```python
from build123d import *

# Parameters (mm, degrees)
F0_R     = 0.5
F1_DEPTH = 9
F2_W     = 3
F2_H     = 2
F3_DEPTH = 1.501


with BuildPart() as f1:
    # F0 (on Right) → F1 (new body)
    with BuildSketch(Plane.YZ):
        with BuildLine():
            ThreePointArc((0, 1.5), (-0.75, 0.75), (0, 0))
            Line((0, 0), (20, 0))
            ThreePointArc((20, 0), (20.75, 0.75), (20, 1.5))
            Line((20, 1.5), (0, 1.5))
        make_face()
        with Locations((0, 0.75)):
            Circle(F0_R, mode=Mode.SUBTRACT)
    extrude(amount=F1_DEPTH)

    # F2 (on Top) → F3 (cut, through all)
    with BuildSketch(Plane.XY):
        with Locations((1.5, 0.25)):
            Rectangle(F2_W, F2_H)
        with Locations((7.5, 0.25)):
            Rectangle(F2_W, F2_H)
    extrude(amount=F3_DEPTH, mode=Mode.SUBTRACT)


solid = f1.part
```
Work out the finished part from the listing and answer in its coordinate system (mm). A direction names the side the tool comes from. Give positions to 0.01 mm unless a question says otherwise; leave off trailing zeros. Loops run counter-clockwise (first coordinate to the right, second up) from the corner with the lowest first, then second, coordinate; pieces in that order, holes last. Notation, with made-up numbers: (-13.5, 83.5) -> (45.5, 83.5) arc R20 cw to (45.5, 100.5) -> close; hole circle Ø5 at (31.25, 11). An arc over 180 degrees is marked (long way). Write item = value, one per line. Start each with the question number.
(1) Find the intervals of material crossed by probe 1 along Y at (x, z) = (4.85, 0.75); probe 2 along Y at (x, z) = (6.25, 0.7); probe 3 along Y at (x, z) = (2.25, 0.35), in increasing order. Write a range as from..to.
(2) Which of the six approach directions +Z, -Z, +X, -X, +Y, -Y give full straight-line access (tool end or side, diameter ignored) to faces 1 (the flat face through (7, 1.25, 1)), 2 (the cylindrical face through (4.44, 20.75, 0.73)), 3 (the flat face through (3, 1, 1))?
(3) Find section A-A on z = 0.75. Give the vertices of the cut face in (x, y).
(4) The mould has two halves that part along Z. Classify faces 4 (the flat face through (6, 1, 1)), 5 (the cylindrical face through (4.479, -0.108, 0.262)), 6 (the flat face through (4, 10, 1.5)): +Z half, -Z half, draft (parallel to the pull), parting line (faces both ways), or undercut.
(5) Find section B-B on x = 2.25. Give the vertices of the cut face in (y, z), and give its area (3 significant figures).
(6) Given pin 1 Ø0.8 at (x, z) = (7, 0.5) entering from -Y; pin 2 Ø0.8 at (y, z) = (0, 1) entering from +X, each flat-ended and moving along its own axis, determine where each tip first touches the part or whether it passes through.
From the geometry:
q1.probe_1 = -0.75..-0.5, 0.5..20.75
q1.probe_2 = 1.25..20.75
q1.probe_3 = 1.25..20.63
q2.face_1 = +Z, -Z, +X, -Y
q2.face_2 = +X, -X, +Y
q2.face_3 = +Z, -Z, -X, -Y
q3.outline = (0, 1.25) -> (3, 1.25) -> (3, 0.5) -> (6, 0.5) -> (6, 1.25) -> (9, 1.25) -> (9, 20.75) -> (0, 20.75) -> close; (3, -0.75) -> (6, -0.75) -> (6, -0.5) -> (3, -0.5) -> close
q4.face_4 = draft
q4.face_5 = undercut
q4.face_6 = +Z half
q5.outline = (1.25, 0) -> (20, 0) arc R0.75 ccw to (20, 1.5) -> (1.25, 1.5) -> close
q5.area = 29.0 mm^2
q6.pin_1 = 1.25
q6.pin_2 = 6
